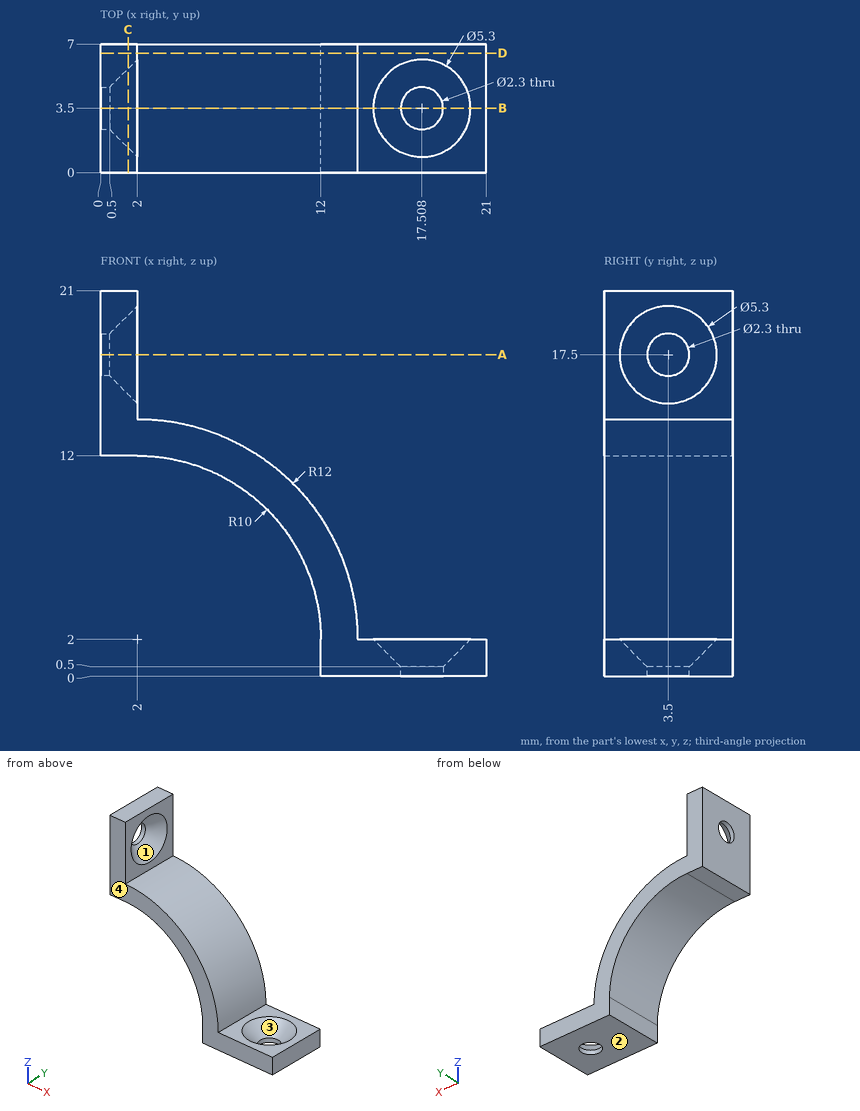
Drawing for the job (mm, zero at the part's lowest x, y, z). Round coordinates to 2 decimals unless told otherwise and drop trailing zeros. Write each loop counter-clockwise with the first axis right and the second up, starting at its lowest first coordinate (ties: lowest second). Pieces come first, ordered by that corner, then holes. Notation, with made-up numbers: M 67.5,-9 L 96.5,-9 A14 ccw 96.5,-1 Z; hole C 52.5,43 d11. An arc over 180 degrees is marked long. Answer as a JSON object with one key per item and string values. Group by question number.
(1) Mould opens along Y. For the marked faces 1, 2, 3 and 4 say: pulls with the +Y half, pulls with the -Y half, needs draft (parallel to the pull), parting line crosses it, or undercut.
(2) Cut at D-D (y = 6.5). Give the cut face in (x, z).
(3) Cut at A-A (z = 17.5). Give the cut face in (x, y).
(4) Cut at B-B (y = 3.5). Give the cut face in (x, z).
(5) Drill centre lines: L1, parallel to Y at x = 0.1, z = 17.5; L2, parallel to X at y = 4.75, z = 20; L3, parallel to Z at x = 1.5, y = 3.5. Where is each one in solid material? Low to high.
(6) Cut at C-C (x = 1.5). Give the cut face in (y, z).
(7) Flat gauge pins, fed straight in: pin 1 (4 mm diameter, centred on x = 5, y = 5, fed in from +Z); pin 2 (4 mm diameter, centred on x = 17.5, y = 1, fed in from +Z); pin 3 (2 mm diameter, centred on x = 0.5, y = 3.5, fed in from -Z). Where does each tip first touch, or does it go through?
Responses:
{
 "1": {"face 1": "undercut", "face 2": "needs draft", "face 3": "undercut", "face 4": "pulls with the -Y half"},
 "2": {"outline": "M 0,12 L 2,12 A10 cw 12,2 L 12,0 L 21,0 L 21,2 L 14,2 A12 ccw 2,14 L 2,21 L 0,21 Z"},
 "3": {"outline": "M 0,0 L 2,0 L 2,0.85 L 0.5,2.35 L 0,2.35 Z; M 0,4.65 L 0.5,4.65 L 2,6.15 L 2,7 L 0,7 Z"},
 "4": {"outline": "M 0,12 L 2,12 A10 cw 12,2 L 12,0 L 16.36,0 L 16.36,0.5 L 14.86,2 L 14,2 A12 ccw 2,14 L 2,14.85 L 0.5,16.35 L 0,16.35 Z; M 0,18.65 L 0.5,18.65 L 2,20.15 L 2,21 L 0,21 Z; M 18.66,0 L 21,0 L 21,2 L 20.16,2 L 18.66,0.5 Z"},
 "5": {"L1": "y = 0 to 2.35, 4.65 to 7", "L2": "x = 0 to 2", "L3": "z = 12 to 15.35, 19.65 to 21"},
 "6": {"outline": "M 0,12 L 7,12 L 7,21 L 0,21 Z; hole C 3.5,17.5 d4.3"},
 "7": {"pin 1": "stops at z = 13.96", "pin 2": "stops at z = 2", "pin 3": "stops at z = 12"}
}
